from build123d import *

# Parameters (mm, degrees)
SKETCH_W     = 95
SKETCH_H     = 36
PAD_DEPTH    = 3
PAD001_DEPTH = 65
SKETCH002_R  = 2
POCKET_DEPTH = 68.001
FILLET_R     = 0.5


with BuildPart() as part:
    # Sketch → Pad (new body)
    with BuildSketch(Plane.YZ):
        with Locations((0, 18)):
            Rectangle(SKETCH_W, SKETCH_H)
    extrude(amount=PAD_DEPTH)

    # Sketch001 (on Face6 of Pad) → Pad001 (join)
    with BuildSketch(Plane.YZ.offset(3)):
        Polygon((-47.5, 0), (-47.5, 3), (-44.3, 3), (-41.3, 6), (-44.3, 9), (-44.3, 12), (-38.3, 12), (-38.3, 3), (38.3, 3), (38.3, 12), (44.3, 12), (44.3, 9), (41.3, 6), (44.3, 3), (47.5, 3), (47.5, 0), align=None)
    extrude(amount=PAD001_DEPTH)

    # Sketch002 (on Face1 of Pad001) → Pocket (cut, through all)
    with BuildSketch(Plane(origin=(0, 0, 0), x_dir=(0, 1, 0), z_dir=(-1, 0, 0))):
        with Locations((-42.5, -18)):
            Circle(SKETCH002_R)
        with Locations((42.5, -18)):
            Circle(SKETCH002_R)
    extrude(amount=-POCKET_DEPTH, mode=Mode.SUBTRACT)

    # Fillet
    fillet_edges = [part.edges().sort_by_distance(p)[0] for p in [
        (0, 0, 0),
        (34, 47.5, 0),
        (68, 0, 0),
        (34, -47.5, 0),
        (0, -47.5, 18),
        (0, 47.5, 18),
        (0, 0, 36),
        (0, 40.5, 18),
        (0, -44.5, 18),
    ]]
    fillet(fillet_edges, radius=FILLET_R)


solid = part.part
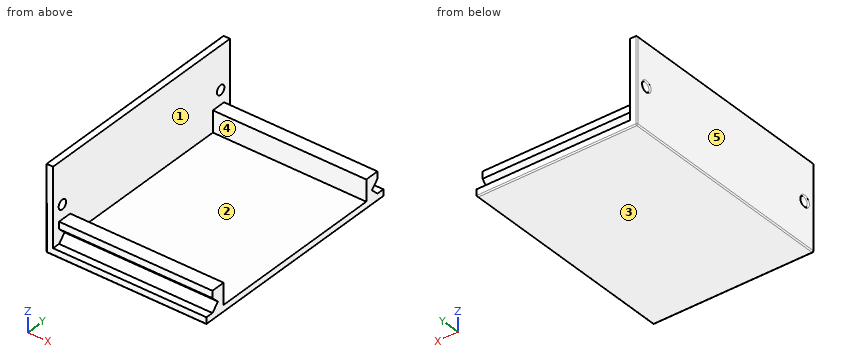
Model file for the job. Use its own axes, mm. Face numbers are marked on the shaded views. A direction names the side the tool comes from. Give positions to 0.01 mm unless a question says otherwise; leave off trailing zeros. Order: outer loops, then holes, each group sorted by start corner. A loop starts at its lowest first (then second) coordinate and runs counter-clockwise, first axis right, second up. Notation, with made-up numbers: (53, -29) - (88, -29) arc R16 cw to (88, -17) - close; hole circle Ø6 at (53, -38). An arc over 180 degrees is marked (long way). Return JSON: item names as keys, results as strings.
1) Flat gauge pins, fed straight in: P1, Ø1, axis at x = 14, z = 13, coming from the -Y side; P2, Ø3.5, axis at x = 28, y = -45.5, coming from the +Z side; P3, Ø8, axis at y = 3, z = 28.5, coming from the +X side; P4, Ø1, axis at x = 39.5, y = 46, coming from the +Z side. Where does each tip first touch, or does it go through?
Geometry says:
{"P1": "through", "P2": "z = 12", "P3": "x = 3", "P4": "z = 3"}
2) Cut at A-A, the plane y = -42.5. Give the cut face in (x, z).
Geometry says:
{"outline": "(0, 0.5) arc R0.5 ccw to (0.5, 0) - (67.5, 0) arc R0.5 ccw to (68, 0.5) - (68, 4.8) - (3, 4.8) - (3, 7.2) - (68, 7.2) - (68, 12) - (3, 12) - (3, 16) - (0.5, 16) arc R0.5 ccw to (0, 15.5) - close; (0, 20.5) arc R0.5 ccw to (0.5, 20) - (3, 20) - (3, 36) - (0.5, 36) arc R0.5 ccw to (0, 35.5) - close"}
3) 3-axis set-ups, long thin cutter, end or side, ignore diameter. For the marked faces 4 and 5: which of +Z, -Z, +X, -X, +Y, -Y reach the whole face in a straight line?
Geometry says:
{"face 4": "+Z, +X", "face 5": "+Z, -Z, -X, +Y, -Y"}
4) Pull direction Y, two halves, no side cores. Call the marked faces 1, 2 and 3: pulls with the +Y half, pulls with the -Y half, needs draft (parallel to the pull), parting line crosses it, or undercut.
Geometry says:
{"face 1": "undercut", "face 2": "undercut", "face 3": "needs draft"}
5) Cut at B-B, the plane z = 18. Give the cut face in (x, y).
Geometry says:
{"outline": "(0, -47) arc R0.5 ccw to (0.5, -47.5) - (3, -47.5) - (3, -44.5) - (0.5, -44.5) arc R0.5 ccw to (0, -45) - close; (0, -40) arc R0.5 ccw to (0.5, -40.5) - (3, -40.5) - (3, 40.5) - (0.5, 40.5) arc R0.5 ccw to (0, 40) - close; (0, 45) arc R0.5 ccw to (0.5, 44.5) - (3, 44.5) - (3, 47.5) - (0.5, 47.5) arc R0.5 ccw to (0, 47) - close"}
6) Cut at D-D, the plane z = 28. Give the cut face in (x, y).
Geometry says:
{"outline": "(0, -47) arc R0.5 ccw to (0.5, -47.5) - (3, -47.5) - (3, 47.5) - (0.5, 47.5) arc R0.5 ccw to (0, 47) - close"}
7) Cut at C-C, the plane x = 15.5. Give the cut face in (y, z).
Geometry says:
{"outline": "(-47.5, 0.5) arc R0.5 ccw to (-47, 0) - (47, 0) arc R0.5 ccw to (47.5, 0.5) - (47.5, 3) - (44.3, 3) - (41.3, 6) - (44.3, 9) - (44.3, 12) - (38.3, 12) - (38.3, 3) - (-38.3, 3) - (-38.3, 12) - (-44.3, 12) - (-44.3, 9) - (-41.3, 6) - (-44.3, 3) - (-47.5, 3) - close"}
8) Probe line 1 (Y direction, x = 2.05, z = 18); line 2 (Z direction, x = 2.55, y = 42.5); line 3 (X direction, y = -2, z = 22). List the from-to ranges inside material, lowest first. Write a range as from..to.
Geometry says:
{"line 1": "-47.5..-44.5, -40.5..40.5, 44.5..47.5", "line 2": "0..16, 20..36", "line 3": "0..3"}
